```python
from build123d import *

# Parameters (mm, degrees)
EXTRUDE_1_DEPTH      = 50
SKETCH_2_R           = 4.999999999999998
CUT_EXTRUDE_1_DEPTH  = 98.87084830229739
SKETCH_3_R           = 15
EXTRUDE_2_DEPTH      = 3
CUT_EXTRUDE_3_REACH  = 108.899
SKETCH_5_R           = 5.000000000000001
SKETCH_6_R           = 5.0000000000000036
CUT_EXTRUDE_5_DEPTH  = 107.89919436089083
CUT_EXTRUDE_7_DEPTH  = 120.99999999999977
CUT_EXTRUDE_10_DEPTH = 10
SKETCH_9_R           = 25
SKETCH_9_R_2         = 15
EXTRUDE_3_DEPTH      = 3
SKETCH_10_R          = 5.0000000000000036
EXTRUDE_4_DEPTH      = 8
SKETCH_11_W          = 70
SKETCH_11_H          = 50.00000000000001
CUT_EXTRUDE_11_DEPTH = 8
SKETCH_12_R          = 25.000000000000004
EXTRUDE_6_DEPTH      = 3
CUT_EXTRUDE_14_DEPTH = 6.500000000000001
SCALE_1_SCALE        = 0.5
SCALE_2_SCALE        = 1.2


with BuildPart() as part:
    # 草图1 → 凸台-拉伸1 (new body)
    with BuildSketch(Plane(origin=(0, 0, 0), x_dir=(1, 0, 0), z_dir=(0, 1, 0))):
        with BuildLine():
            Line((-23.323422211177558, 7.232068902691513), (-23.323422211177558, 70))
            Line((-23.323422211177558, 70), (46.67657778882245, 70))
            add(Edge.make_bspline(
                [(46.67657778882245, 70), (-25.880344692728325, -52.054397164609135), (-23.323422211177558, 7.232068902691513)],
                knots=[0, 0, 0, 1, 1, 1], degree=2))
        make_face()
    extrude(amount=EXTRUDE_1_DEPTH)

    # 草图2 → 切除-拉伸1 (cut, through all)
    with BuildSketch(Plane(origin=(0, 50, 0), x_dir=(1, 0, 0), z_dir=(0, 1, 0))):
        with Locations(Location((-14.323422211177558, -0.8457019663808466, 0), (0, 0, 270))):
            Circle(SKETCH_2_R)
    extrude(amount=-CUT_EXTRUDE_1_DEPTH, mode=Mode.SUBTRACT)

    # 草图3 → 凸台-拉伸2 (add)
    with BuildSketch(Plane(origin=(0, 0, -70), x_dir=(-1, 0, 0), z_dir=(0, 0, -1))):
        with Locations(Location((-21.676577788822446, 25, 0), (0, 0, 180))):
            Circle(SKETCH_3_R)
    extrude(amount=EXTRUDE_2_DEPTH)

    # 草图5 → 切除-拉伸3 (cut, up to next)
    with BuildSketch(Plane(origin=(0, 0, -70), x_dir=(-1, 0, 0), z_dir=(0, 0, -1)), mode=Mode.PRIVATE) as cut_extrude_3_sk1:
        with Locations((-21.676577788822446, 25)):
            Circle(SKETCH_5_R)
    cut_extrude_3_tool1 = extrude(cut_extrude_3_sk1.sketch, amount=-CUT_EXTRUDE_3_REACH, mode=Mode.PRIVATE) & part.part
    add(cut_extrude_3_tool1.solids().sort_by_distance((21.676578, 25, -70))[0], mode=Mode.SUBTRACT)

    # 草图6 → 切除-拉伸5 (cut, through all)
    with BuildSketch(Plane.XY.offset(-70)):
        with Locations(Location((21.676577788822446, 25, 0), (0, 0, 180))):
            Circle(SKETCH_6_R)
    extrude(amount=-CUT_EXTRUDE_5_DEPTH, mode=Mode.SUBTRACT)

    # 草图7 → 切除-拉伸7 (cut)
    with BuildSketch(Plane.ZY.offset(23.323422211177558)):
        Polygon((-65.00000000000001, 47), (34.99999999999999, 47), (34.99999999999999, 3.0000000000000027), (-65.00000000000001, 3.0000000000000018), align=None)
    extrude(amount=-CUT_EXTRUDE_7_DEPTH, mode=Mode.SUBTRACT)

    # 草图8 → 切除-拉伸10 (cut)
    with BuildSketch(Plane(origin=(-23.323422211177558, 0, 0), x_dir=(0, 0, -1), z_dir=(1, 0, 0))):
        Polygon((7.232068902691513, 3.0000000000000027), (7.232068902691513, 47), (4.887844e-11, 47), (4.887757e-11, 3.000000000000002), align=None)
    extrude(amount=-CUT_EXTRUDE_10_DEPTH, mode=Mode.SUBTRACT)

    # 草图9 → 凸台-拉伸3 (add)
    with BuildSketch(Plane(origin=(0, 0, -70), x_dir=(-1, 0, 0), z_dir=(0, 0, -1))):
        with Locations(Location((-21.676577788822446, 25, 0), (0, 0, 180))):
            Circle(SKETCH_9_R)
        with Locations((-21.676577788822446, 25)):
            Circle(SKETCH_9_R_2, mode=Mode.SUBTRACT)
    extrude(amount=EXTRUDE_3_DEPTH)

    # 草图10 → 凸台-拉伸4 (add)
    with BuildSketch(Plane(origin=(0, 0, -73.00000000000001), x_dir=(-1, 0, 0), z_dir=(0, 0, -1))):
        with Locations((-21.676577788822446, 25)):
            Circle(SKETCH_10_R)
    extrude(amount=-EXTRUDE_4_DEPTH)

    # 草图11 → 切除-拉伸11 (cut)
    with BuildSketch(Plane(origin=(0, 0, -70), x_dir=(-1, 0, 0), z_dir=(0, 0, -1))):
        with Locations((-11.676577788822447, 25.000000000000004)):
            Rectangle(SKETCH_11_W, SKETCH_11_H)
    extrude(amount=CUT_EXTRUDE_11_DEPTH, mode=Mode.SUBTRACT)

    # 草图12 → 凸台-拉伸6 (add)
    with BuildSketch(Plane(origin=(0, 0, -70), x_dir=(-1, 0, 0), z_dir=(0, 0, -1))):
        with Locations(Location((-11.676577788822453, 25.000000000000004, 0), (0, 0, 270))):
            Circle(SKETCH_12_R)
    extrude(amount=EXTRUDE_6_DEPTH)

    # 草图19 → 切除-拉伸14 (cut, symmetric)
    with BuildSketch(Plane(origin=(0, 0, -70), x_dir=(-1, 0, 0), z_dir=(0, 0, -1))):
        with BuildLine():
            ThreePointArc((-7.607910432788657, 27.906190968595336), (-11.676577788822362, 30.000000000000004), (-15.745245144856133, 27.90619096859546))
            Line((-15.745245144856124, 27.90619096859548), (-11.676577788822456, 25.000000000000004))
            Line((-11.676577788822442, 25), (-7.607910432788756, 27.90619096859549))
        make_face()
        with BuildLine():
            Line((-11.676577788822456, 25.000000000000004), (-15.745245144856124, 27.90619096859548))
            ThreePointArc((-15.745245144856133, 27.90619096859546), (-16.67657778882244, 25), (-15.745245144856128, 22.09380903140454))
            Line((-15.745245144856106, 22.093809031404525), (-11.676577788822442, 25))
        make_face()
        with BuildLine():
            Line((-7.607910432788756, 27.90619096859549), (-11.676577788822442, 25))
            Line((-11.676577788822456, 25.000000000000004), (-7.607910432788778, 22.09380903140452))
            ThreePointArc((-7.607910432788663, 22.09380903140466), (-6.915100246075392, 23.47411284496017), (-6.676577788822438, 25.000000000000004))
            ThreePointArc((-6.676577788822438, 25.000000000000004), (-6.915100246075391, 26.525887155039833), (-7.607910432788657, 27.906190968595336))
        make_face()
        with BuildLine():
            Line((-7.607910432788778, 22.09380903140452), (-11.676577788822456, 25.000000000000004))
            Line((-11.676577788822442, 25), (-15.745245144856106, 22.093809031404525))
            ThreePointArc((-15.745245144856128, 22.09380903140454), (-11.676577788822364, 20.000000000000004), (-7.607910432788663, 22.09380903140466))
        make_face()
    extrude(amount=CUT_EXTRUDE_14_DEPTH, both=True, mode=Mode.SUBTRACT)


with BuildPart() as part_1:
    # 缩放比例1: scaled about (6.493831083, 24.99994197, -53.778737611)
    add(part.part.scale(SCALE_1_SCALE).moved(Location((3.2469155415, 12.499970985, -26.8893688055))))


with BuildPart() as part_2:
    # 缩放比例2: scaled about (6.493831083, 24.99994197, -53.778737611)
    add(part_1.part.scale(SCALE_2_SCALE).moved(Location((-1.2987662165999998, -4.999988393999999, 10.755747522199997))))


solid = part_2.part
```
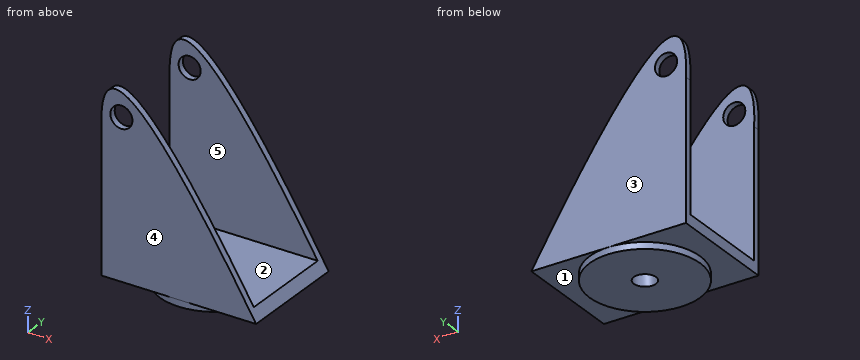
Work out the finished part from the listing and answer in its coordinate system (mm). Face numbers are marked on the shaded views. A direction names the side the tool comes from. Coordinates: 2 decimals unless noted, no trailing zeros. Answer as a JSON object with one key per item and string values.
1. Each of these flat-tipped pins is pushed along its axis until it touches: P1, Ø5.5, axis at x = -6, z = -21, coming from the -Y side; P2, Ø12, axis at x = 15.5, y = 27.5, coming from the +Z side. Where does it stop, or does it pass through?
Output values:
{"P1": "passes through", "P2": "stops at z = -60.51"}
2. Consider line 1 (Y direction, x = -1.5, z = -37.5); line 2 (Z direction, x = 4, y = 14); line 3 (Z direction, x = -6, y = 34.5). Determine where each line is inside the solid, lowest interval first.
Output values:
{"line 1": "y = 10 to 11.8, 38.2 to 40", "line 2": "z = -65.31 to -60.51", "line 3": "z = -63.51 to -60.51"}
3. A tool of negligible diameter and unlimited length cuts with its end or side. For the marked faces 4 and 5, from which of +Z, -Z, +X, -X, +Y, -Y can it reach the whole face along a straight path? Write none if from no direction.
Output values:
{"face 4": "+Z, -Z, +X, -X, -Y", "face 5": "+Z, +X, -X"}
4. The mould has two halves that part along Y. Classify the marked faces 1, 2 and 3: +Y half, -Y half, draft (parallel to the pull), parting line (faces both ways), or undercut.
Output values:
{"face 1": "draft", "face 2": "undercut", "face 3": "+Y half"}
